For this review, take the finished solid that the model builds, in its own axes (mm). A direction names the side the tool comes from. Coordinates: 2 decimals unless noted, no trailing zeros. Loops run counter-clockwise (first coordinate to the right, second up) from the corner with the lowest first, then second, coordinate; pieces in that order, holes last. Notation, with made-up numbers: M 16,78.5 L 23,78.5 A35 ccw 23,114.5 Z; hole C 79.5,28 d4. An arc over 180 degrees is marked long. Use one line per item in the form item = value.
Autodesk Inventor part; units mm, degrees
ref_plane "YZ Plane" through (0, 0, 0) normal (1, 0, 0) x (0, 1, 0)
ref_plane "XZ Plane" through (0, 0, 0) normal (0, 1, 0) x (-1, 0, 0)
ref_plane "XY Plane" through (0, 0, 0) normal (0, 0, 1) x (1, 0, 0)
sketch "スケッチ1" plane through (0, 0, 0) normal (0, 0, 1) x (1, 0, 0)
  circle A0 centre (0, 0) radius 9
  circle A1 centre (0, 0) radius 6
  dimension "d0" = 18
  dimension "d1" = 12
extrude "押し出し1" add sketch "スケッチ1" along normal blind 1
sketch "スケッチ2" plane through (0, 0, 1) normal (0, 0, 1) x (1, 0, 0)
  circle A0 centre (0, 0) radius 9
  circle A1 centre (0, 0) radius 6
  circle A2 centre (0, 0) radius 7
  dimension "d4" = 14
extrude "押し出し2" add sketch "スケッチ2" along normal blind 5 contours A2
chamfer "面取り1" distance 0.5 angle 45 1 edges at (-7, 0, 6)
properties part number "オイレスw5f6-10a" material "アセタール樹脂、黒"
1. Tool access review of faces 1 (the face through (0, -7.3, 1)), 2 (the face through (2, -6, 0)): name each direction out of +Z, -Z, +X, -X, +Y, -Y from which nothing blocks a thin tool from reaching the whole face with its end or side.
Computed values:
face_1 = +Z
face_2 = -Z, +X, -X, +Y, -Y
2. Wall thickness on line 1 along Y through (x, z) = (0, 3.15); line 2 along X through (y, z) = (4.75, 1.2); line 3 along Z through (x, y) = (5.25, -6.75): over which ranges is each line inside the solid? List them lowest first. Write a range as from..to.
Computed values:
line_1 = -7..-6, 6..7
line_2 = -5.14..-3.67, 3.67..5.14
line_3 = 0..1
3. For pin 1 Ø1 at (x, y) = (4, -7) entering from -Z; pin 2 Ø1 at (x, z) = (-3.5, 1) entering from -Y, all flat-tipped, find the tip position at first contact; note any pin that passes through.
Computed values:
pin_1 = 0
pin_2 = -8.49
4. Consider section C-C on z = 1.45. Write out the cut boundary in (x, y).
Computed values:
outline = C 0,0 d14; hole C 0,0 d12
5. Consider section A-A on x = 0. Write out the cut boundary in (y, z).
Computed values:
outline = M -9,0 L -6,0 L -6,6 L -6.5,6 L -7,5.5 L -7,1 L -9,1 Z; M 6,0 L 9,0 L 9,1 L 7,1 L 7,5.5 L 6.5,6 L 6,6 Z
6. Draft analysis for pull direction X (two halves, no side actions). For faces 3 (the face through (-6, 0, 3)), 4 (the face through (2, -6, 6)), 5 (the face through (6.466, 2.681, 3.218)), state which applies: +X half, -X half, draft (parallel to the pull), parting line (faces both ways), or undercut.
Computed values:
face_3 = undercut
face_4 = draft
face_5 = parting line
